Input: part model. Units: mm. Frame: model coordinates. Coordinates: 2 decimals unless noted, no trailing zeros. Loops run counter-clockwise (first coordinate to the right, second up) from the corner with the lowest first, then second, coordinate; pieces in that order, holes last.
Item 1: Section C-C on y = 59. Return loops of the section in (x, z).
Item 2: Section B-B on x = 74.5. Return loops of the section in (y, z), and give its area (3 significant figures).
Item 3: Ray query, line 1 along X through (y, z) = (-63.5, 5.25); line 2 along Y through (x, z) = (-89.5, 3.25); line 3 along Y through (x, z) = (-89, 1.25). Return the intervals inside material, ascending.
Item 4: Section A-A on z = 4.75. Return loops of the section in (x, y).
Autodesk Inventor part; units mm, degrees
ref_plane "YZ Plane" through (0, 0, 0) normal (1, 0, 0) x (0, 1, 0)
ref_plane "XZ Plane" through (0, 0, 0) normal (0, 1, 0) x (-1, 0, 0)
ref_plane "XY Plane" through (0, 0, 0) normal (0, 0, 1) x (1, 0, 0)
sketch "Эскиз1" plane through (0, 0, 0) normal (0, 0, 1) x (1, 0, 0)
  line L0 (11.0194, 105.4233) -> (11.0194, 99.2429)
  line L1 (11.0194, 99.2429) -> (-11.0194, 99.2429)
  line L2 (-11.0194, 99.2429) -> (-11.0194, 105.4233)
  line L3 (-11.0194, 105.4233) -> (11.0194, 105.4233)
  circle A0 centre (104, 76) radius 1.481
  circle A1 centre (104, -76) radius 1.481
  circle A2 centre (-104, -76) radius 1.481
  circle A3 centre (-104, 76) radius 1.481
  arc A4 (135.5, -107) -> (137.5, -105) centre (135.5, -105) ccw
  line L4 (137.5, 105) -> (137.5, -105)
  arc A5 (137.5, 105) -> (135.5, 107) centre (135.5, 105) ccw
  line L5 (-135.5, 107) -> (135.5, 107)
  arc A6 (-135.5, 107) -> (-137.5, 105) centre (-135.5, 105) ccw
  line L6 (-137.5, -105) -> (-137.5, 105)
  arc A7 (-137.5, -105) -> (-135.5, -107) centre (-135.5, -105) ccw
  line L7 (135.5, -107) -> (-135.5, -107)
  line L8 (-132.5, -102) -> (-132.5, 102)
  line L9 (-132.5, 102) -> (132.5, 102)
  line L10 (132.5, 102) -> (132.5, -102)
  line L11 (132.5, -102) -> (-132.5, -102)
  point P0 (0, 0)
  dimension "d0" = 5
extrude "Выдавливание1" add sketch "Эскиз1" along normal blind 7 contours L9 L10 L11 L8 L2 L1 L0 | L0 L1 L2 L9
sketch "Эскиз2" plane through (0, 0, 7) normal (0, 0, 1) x (1, 0, 0)
  line L0 (-146.9193, 158.9761) -> (149.0915, 158.9761) construction
  line L1 (149.0915, 158.9761) -> (149.0915, -137.0348) construction
  line L2 (149.0915, -137.0348) -> (-146.9193, -137.0348) construction
  line L3 (-146.9193, -137.0348) -> (-146.9193, 158.9761) construction
  point P0 (0, 0)
decal "Маркировка1"
sketch "Эскиз4" plane through (0, 0, 0) normal (0, 0, -1) x (-1, 0, 0)
  line L0 (-100, 90) -> (100, 90)
  line L1 (100, 90) -> (100, -90)
  line L2 (100, -90) -> (-100, -90)
  line L3 (-100, -90) -> (-100, 90)
  line L4 (-100, 90) -> (100, -90) construction
  line L5 (100, 90) -> (-100, -90) construction
  line L6 (100, -55) -> (65, -90)
  line L7 (-65, -90) -> (-100, -55)
  line L8 (-100, 55) -> (-65, 90)
  line L9 (100, 55) -> (65, 90)
  line L10 (-65, 90) -> (65, 90) construction
  line L11 (65, 90) -> (65, -90) construction
  line L12 (65, -90) -> (-65, -90) construction
  line L13 (-65, -90) -> (-65, 90) construction
  line L14 (-65, 90) -> (65, -90) construction
  line L15 (65, 90) -> (-65, -90) construction
  line L16 (-276.1466, 193.443) -> (276.1466, 193.443)
  line L17 (276.1466, 193.443) -> (276.1466, -193.443)
  line L18 (276.1466, -193.443) -> (-276.1466, -193.443)
  line L19 (-276.1466, -193.443) -> (-276.1466, 193.443)
  line L20 (-276.1466, 193.443) -> (276.1466, -193.443) construction
  line L21 (276.1466, 193.443) -> (-276.1466, -193.443) construction
  point P0 (0, 0)
  point P1 (0, 0)
  dimension "d18" = 200
  dimension "d19" = 180
  dimension "d20" = 45
  dimension "d21" = 45
  dimension "d22" = 45
  dimension "d23" = 45
  dimension "d24" = 130
extrude "Выдавливание3" cut sketch "Эскиз4" against normal blind 10 contours L0 L8 L3 | L0 L1 L9 | L7 L2 L3 | L1 L2 L6 | L16 L17 L18 L19
properties part number "утепление стола"
Results found:
1. outline: (-96, 0) - (96, 0) - (96, 7) - (-96, 7) - close
2. outline: (-80.5, 0) - (80.5, 0) - (80.5, 7) - (-80.5, 7) - close
2. area: 1,130 mm2
3. line 1: x = -91.5 to 91.5
3. line 2: y = -65.5 to 65.5
3. line 3: y = -66 to 66
4. outline: (-100, -55) - (-65, -90) - (65, -90) - (100, -55) - (100, 55) - (65, 90) - (-65, 90) - (-100, 55) - close
